For this review, take the finished solid that the model builds, in its own axes (mm). A direction names the side the tool comes from. Coordinates: 2 decimals unless noted, no trailing zeros. Order: outer loops, then holes, each group sorted by start corner. A loop starts at its lowest first (then second) coordinate and runs counter-clockwise, first axis right, second up. Notation, with made-up numbers: (34.5, 38) - (73.5, 38) arc R4 ccw to (73.5, 44) - close; hole circle Ø2 at (-12, 12). An arc over 180 degrees is marked (long way). One line per item, written item: value. Start each with the question number.
(1) Consider section C-C on z = 9. Write out the cut boundary in (x, y).
(2) Consider section A-A on y = -44.45. Write out the cut boundary in (x, z), then the cut area to 3 significant figures.
(3) Mouldability with a two-part tool opening along Z and no side actions: class faces 1 (the cylindrical face through (-22.448, -6.439, 18.175)), 2 (the flat face through (-44.12, -12, -1)), 3 (the flat face through (-7, -29, -21.722)), 4 (the cylindrical face through (25.641, -34.372, 18.175)) as released by +Z, released by -Z, zero draft, split by the parting line, or undercut.
(4) Consider section D-D on x = 13.5. Write out the cut boundary in (y, z), then the cut area to 3 significant figures.
(5) Clearance check with flat-ended pins moving along their axes: pin 1 (2 mm diameter, centred on x = -5, z = 45.5, fed in from -Y); pin 2 (17 mm diameter, centred on y = -41.5, z = 29, fed in from -X); pin 3 (4 mm diameter, centred on x = -8, y = -25.5, fed in from +Z). State where each tip first meets the part, or that it passes through.
(6) Consider section B-B on x = -4.5. Write out the cut boundary in (y, z), then the cut area to 3 significant figures.
(7) For faces 5 (the flat face through (-1, -76.2, -3)), 6 (the flat face through (-13, -31, -2.672)), list the 3-axis set-ups (+Z, -Z, +X, -X, +Y, -Y) from which the entire face can be reached by the end or side of a thin tool; tool diameter is ignored.
(8) To check wall thickness, follow line 1 along Z through (x, y) = (27, -44); line 2 along Y through (x, z) = (2, 1.5); line 3 along X through (y, z) = (-56, 12.5). State the ranges of each line that lie inside material, in increasing order.
```python
from build123d import *

# Parameters (mm, degrees)
F0_W     = 76.2
F0_H     = 76.2
F1_DEPTH = 76.2
F2_W     = 63.5
F2_H     = 57.15
F3_DEPTH = 63.5
F5_R     = 12.7
F7_DEPTH = 25.4
F6_R     = 12.7
F8_DEPTH = 25.4
F4_R     = 12.7
F9_DEPTH = 25.4


with BuildPart() as f1:
    # F0 (on Front) → F1 (new body)
    with BuildSketch(Plane.XZ):
        with Locations((-6.020044, 16.377596)):
            Rectangle(F0_W, F0_H)
    extrude(amount=F1_DEPTH)

    # F2 (on face) → F3 (cut)
    with BuildSketch(Plane.XZ.offset(76.2)):
        with Locations((-12.370044, 25.902596)):
            Rectangle(F2_W, F2_H)
    extrude(amount=-F3_DEPTH, mode=Mode.SUBTRACT)

    # F5 (on face) → F7 (cut)
    with BuildSketch(Plane(origin=(19.379956, 0, 0), x_dir=(0, -1, 0), z_dir=(-1, 0, 0))):
        with Locations((44.45, 25.902596)):
            Circle(F5_R)
    extrude(amount=-F7_DEPTH, mode=Mode.SUBTRACT)

    # F6 (on face) → F8 (cut)
    with BuildSketch(Plane.XZ.offset(12.7)):
        with Locations((-12.370044, 25.902596)):
            Circle(F6_R)
    extrude(amount=-F8_DEPTH, mode=Mode.SUBTRACT)

    # F4 (on face) → F9 (cut)
    with BuildSketch(Plane.XY.offset(-2.672404)):
        with Locations((-12.370044, -44.45)):
            Circle(F4_R)
    extrude(amount=-F9_DEPTH, mode=Mode.SUBTRACT)


solid = f1.part
```
Geometry check:
1. outline: (-44.12, -12.7) - (19.38, -12.7) - (19.38, -76.2) - (32.08, -76.2) - (32.08, 0) - (-44.12, 0) - close
2. outline: (-44.12, -21.72) - (-25.07, -21.72) - (-25.07, -2.67) - (-44.12, -2.67) - close; (0.33, -21.72) - (32.08, -21.72) - (32.08, 13.2) - (19.38, 13.2) - (19.38, -2.67) - (0.33, -2.67) - close; (19.38, 38.6) - (32.08, 38.6) - (32.08, 54.48) - (19.38, 54.48) - close
2. area: 1,370 mm^2
3. face 1: undercut
3. face 2: zero draft
3. face 3: released by -Z
3. face 4: undercut
4. outline: (-76.2, -21.72) - (0, -21.72) - (0, 54.48) - (-12.7, 54.48) - (-12.7, -2.67) - (-76.2, -2.67) - close
4. area: 2,180 mm^2
5. pin 1: stops at y = -12.7
5. pin 2: stops at x = 19.38
5. pin 3: stops at z = -2.67
6. outline: (-76.2, -21.72) - (-54.42, -21.72) - (-54.42, -2.67) - (-76.2, -2.67) - close; (-34.48, -21.72) - (0, -21.72) - (0, 15.94) - (-12.7, 15.94) - (-12.7, -2.67) - (-34.48, -2.67) - close; (-12.7, 35.87) - (0, 35.87) - (0, 54.48) - (-12.7, 54.48) - close
6. area: 1,540 mm^2
7. face 5: +Z, -Z, +X, -X, -Y
7. face 6: +Z, -X, -Y
8. line 1: z = -21.72 to 13.21, 38.59 to 54.48
8. line 2: y = -12.7 to 0
8. line 3: x = 19.38 to 32.08
